```python
from build123d import *

# Parameters (mm, degrees)
SKETCH_1_R          = 2.2
SKETCH_1_R_2        = 2.25
EXTRUDE_1_DEPTH     = 2
EXTRUDE_START       = -2
EXTRUDE_2_DEPTH     = 2
SKETCH_3_R          = 2.25
CUT_EXTRUDE_1_DEPTH = 23
SKETCH_3_3_R        = 2.25
EXTRUDE_3_DEPTH     = 2
SKETCH_5_W          = 104
SKETCH_5_H          = 6
CUT_EXTRUDE_2_DEPTH = 24
FILLET_1_R          = 6


with BuildPart() as part:
    # Sketch 1 → Extrude 1 (new body)
    with BuildSketch(Plane.XY):
        with BuildLine():
            Line((63, 28), (-63, 28))
            ThreePointArc((-63, 28), (-64.414213562, 27.414213562), (-65, 26))
            Line((-65, 26), (-65, -26))
            ThreePointArc((-65, -26), (-64.414213562, -27.414213562), (-63, -28))
            Line((-63, -28), (-54, -28))
            ThreePointArc((-54, -28), (-52.585786438, -27.414213562), (-52, -26))
            Line((-52, -26), (-52, -8))
            ThreePointArc((-52, -8), (-51.414213562, -6.585786438), (-50, -6))
            Line((-50, -6), (50, -6))
            ThreePointArc((50, -6), (51.414213562, -6.585786438), (52, -8))
            Line((52, -8), (52, -26))
            ThreePointArc((52, -26), (52.585786438, -27.414213562), (54, -28))
            Line((54, -28), (63, -28))
            ThreePointArc((63, -28), (64.414213562, -27.414213562), (65, -26))
            Line((65, -26), (65, 26))
            ThreePointArc((65, 26), (64.414213562, 27.414213562), (63, 28))
        make_face()
        with Locations((-57.5, -9.5)):
            Circle(SKETCH_1_R, mode=Mode.SUBTRACT)
        with Locations((-57.5, 20.5)):
            Circle(SKETCH_1_R, mode=Mode.SUBTRACT)
        with Locations((19.25, 20.5)):
            Circle(SKETCH_1_R, mode=Mode.SUBTRACT)
        with Locations((-19.25, 20.5)):
            Circle(SKETCH_1_R, mode=Mode.SUBTRACT)
        with Locations((57.5, 20.5)):
            Circle(SKETCH_1_R, mode=Mode.SUBTRACT)
        with Locations((57.5, -9.5)):
            Circle(SKETCH_1_R, mode=Mode.SUBTRACT)
        with Locations((27, 2.5)):
            Circle(SKETCH_1_R_2, mode=Mode.SUBTRACT)
        with Locations((-27, 2.5)):
            Circle(SKETCH_1_R_2, mode=Mode.SUBTRACT)
        with BuildLine():
            Line((27.25, 18), (49.5, 18))
            ThreePointArc((49.5, 18), (52, 20.5), (49.5, 23))
            Line((49.5, 23), (27.25, 23))
            ThreePointArc((27.25, 23), (24.75, 20.5), (27.25, 18))
        make_face(mode=Mode.SUBTRACT)
        with BuildLine():
            Line((-11.25, 18), (11, 18))
            ThreePointArc((11, 18), (13.5, 20.5), (11, 23))
            Line((11, 23), (-11.25, 23))
            ThreePointArc((-11.25, 23), (-13.75, 20.5), (-11.25, 18))
        make_face(mode=Mode.SUBTRACT)
        with BuildLine():
            Line((-49.5, 18), (-27.25, 18))
            ThreePointArc((-27.25, 18), (-24.75, 20.5), (-27.25, 23))
            Line((-27.25, 23), (-49.5, 23))
            ThreePointArc((-49.5, 23), (-52, 20.5), (-49.5, 18))
        make_face(mode=Mode.SUBTRACT)
    extrude(amount=EXTRUDE_1_DEPTH)

    # Sketch 2 → Extrude 2 (add)
    with BuildSketch(Plane.XY.offset(2).offset(EXTRUDE_START)):
        with BuildLine():
            Line((-52, -8), (-52, -11))
            Line((-52, -11), (52, -11))
            Line((52, -11), (52, -8))
            ThreePointArc((52, -8), (51.414213562, -6.585786438), (50, -6))
            Line((50, -6), (-50, -6))
            ThreePointArc((-50, -6), (-51.414213562, -6.585786438), (-52, -8))
        make_face()
    extrude(amount=EXTRUDE_2_DEPTH)

    # Sketch 3 → Cut-Extrude 1 (cut)
    with BuildSketch(Plane.XY.offset(2)):
        with BuildLine():
            ThreePointArc((-27, 10.25), (-28.590990258, 9.590990258), (-29.25, 8))
            Line((-29.25, 8), (-27, 8))
            Line((-27, 8), (-27, 10.25))
        make_face()
        with BuildLine():
            Line((-27, 8), (-29.25, 8))
            ThreePointArc((-29.25, 8), (-28.590990258, 6.409009742), (-27, 5.75))
            Line((-27, 5.75), (-27, 8))
        make_face()
        with BuildLine():
            Line((-27, 10.25), (-27, 8))
            Line((-27, 8), (-24.75, 8))
            ThreePointArc((-24.75, 8), (-25.409009742, 9.590990258), (-27, 10.25))
        make_face()
        with BuildLine():
            Line((-24.75, 8), (-27, 8))
            Line((-27, 8), (-27, 5.75))
            ThreePointArc((-27, 5.75), (-25.409009742, 6.409009742), (-24.75, 8))
        make_face()
        with Locations((27, 8)):
            Circle(SKETCH_3_R)
    extrude(amount=-CUT_EXTRUDE_1_DEPTH, mode=Mode.SUBTRACT)

    # Sketch 3_3 → Extrude 3 (add)
    with BuildSketch(Plane.XY.offset(2).offset(EXTRUDE_START)):
        with Locations((27, 2.5)):
            Circle(SKETCH_3_3_R)
        with Locations((-27, 2.5)):
            Circle(SKETCH_3_3_R)
    extrude(amount=EXTRUDE_3_DEPTH)

    # Sketch 5 → Cut-Extrude 2 (cut)
    with BuildSketch(Plane.XY.offset(2)):
        with Locations((0, -8)):
            Rectangle(SKETCH_5_W, SKETCH_5_H)
    extrude(amount=-CUT_EXTRUDE_2_DEPTH, mode=Mode.SUBTRACT)

    # Fillet 1
    fillet_1_edges = [part.edges().sort_by_distance(p)[0] for p in [
        (-52, -5, 1),
        (52, -5, 1),
    ]]
    fillet(fillet_1_edges, radius=FILLET_1_R)


solid = part.part
```
Design review of the part built by this model. Coordinates are the model's own, in mm. A direction names the side the tool comes from. Coordinates: 2 decimals unless noted, no trailing zeros. Loops run counter-clockwise (first coordinate to the right, second up) from the corner with the lowest first, then second, coordinate; pieces in that order, holes last. Notation, with made-up numbers: (82, 45.25) -> (88, 45.25) arc R8 cw to (88, 59.25) -> close; hole circle Ø11 at (-1, 25.5). An arc over 180 degrees is marked (long way). Answer as a JSON object with one key per item and string values.
Q1. The part is to be moulded in two halves that separate along Y. For faces 4 (the flat face through (-1, 7, 0)), 5 (the cylindrical face through (-55.4, -8.84, 0.99)), 6 (the cylindrical face through (28.21, 9.897, 1.014)), 7 (the cylindrical face through (50.289, -6.804, 0.986)), say which applies: +Y half, -Y half, draft (parallel to the pull), parting line (faces both ways), or undercut.
Answer block:
{"face 4": "draft", "face 5": "undercut", "face 6": "undercut", "face 7": "-Y half"}
Q2. Clearance check with flat-ended pins moving along their axes: pin 1 Ø2.5 at (x, y) = (-57.5, 20.5) entering from -Z; pin 2 Ø1 at (x, z) = (-2.5, 0.5) entering from -Y. State where each tip first meets the part, or that it passes through.
Answer block:
{"pin 1": "passes through", "pin 2": "stops at y = -5"}
Q3. To check wall thickness, follow L1, parallel to Y at x = 57.5, z = 1.55; L2, parallel to Y at x = 27, z = 0.6; L3, parallel to Y at x = -46, z = 1.45. State the ranges of each line that lie inside material, in increasing order.
Answer block:
{"L1": "y = -28 to -11.7, -7.3 to 18.3, 22.7 to 28", "L2": "y = -5 to 5.75, 10.25 to 18.01, 22.99 to 28", "L3": "y = -5 to 18, 23 to 28"}
Q4. Take a section at B-B on y = 20.5. Give the number of separate pieces and of enclosed holes in the cut face, plus the area to 3 significant figures.
Answer block:
{"separate pieces": "8", "enclosed holes": "0", "area": "61.3 mm^2"}
Q5. Take a section at A-A on x = -8.5. Give the boundary of the cut face in (y, z).
Answer block:
{"outline": "(-5, 0) -> (18, 0) -> (18, 2) -> (-5, 2) -> close; (23, 0) -> (28, 0) -> (28, 2) -> (23, 2) -> close"}
Q6. Take a section at C-C on y = -14. Give the boundary of the cut face in (x, z), plus the area to 3 significant figures.
Answer block:
{"outline": "(-65, 0) -> (-52, 0) -> (-52, 2) -> (-65, 2) -> close; (52, 0) -> (65, 0) -> (65, 2) -> (52, 2) -> close", "area": "52.0 mm^2"}
Q7. Tool access review of faces 1 (the cylindrical face through (-50.196, -6.711, 0.986)), 2 (the flat face through (-1, 7, 2)), 3 (the cylindrical face through (-52, 20.6, 1)): name each direction out of +Z, -Z, +X, -X, +Y, -Y from which nothing blocks a thin tool from reaching the whole face with its end or side.
Answer block:
{"face 1": "+Z, -Z, -Y", "face 2": "+Z, +X, -X, +Y, -Y", "face 3": "+Z, -Z"}
